Check sheet for the modelled part. Datum: model origin and axes. Units: mm. A direction names the side the tool comes from. Give positions to 0.01 mm unless a question says otherwise; leave off trailing zeros. Order: outer loops, then holes, each group sorted by start corner. A loop starts at its lowest first (then second) coordinate and runs counter-clockwise, first axis right, second up.
Item 1: Gauge pin test, flat ends, axial feed: P1, Ø8, axis at y = -17.5, z = -8, coming from the +X side; P2, Ø6, axis at x = 14, z = -8.5, coming from the -Y side; P3, Ø9, axis at y = -22, z = -4.5, coming from the -X side; P4, Ø12, axis at y = -4.5, z = -23.5, coming from the +X side. Record the tip position at first contact, or that the pin passes through.
Item 2: Material ranges on line 1 along X through (y, z) = (0.15, -20.25); line 2 along Z through (x, y) = (-21, -21.75); line 3 along Z through (x, y) = (-20, -7), recorded low to high.
Item 3: Release check for a two-part mould opening along Z. For faces 4 (the flat face through (-29, -6, -14.6)), 5 (the flat face through (11.719, -8, -48)), 6 (the flat face through (7.804, -5.144, -38.064)) record: released by +Z, released by -Z, zero draft, split by the parting line, or undercut.
Item 4: Sectioned sample at A-A on z = -9.5. Record the boundary of the cut face in (x, y), and give its area (3 significant figures).
Item 5: Sectioned sample at C-C on z = -15.5. Record the boundary of the cut face in (x, y), and give its area (3 significant figures).
Item 6: Access from +Z, -Z, +X, -X, +Y, -Y to the whole of each face (thin tool, end or side, straight path). Record for faces 1 (the flat face through (-3.889, -6, -43)), 2 (the cylindrical face through (-19.17, -16.55, -12.85)), 3 (the flat face through (7.62, -8.4, -48.9)).
Item 7: Sectioned sample at B-B on x = -7.5. Record the boundary of the cut face in (y, z).
from build123d import *

# Parameters (mm, degrees)
EXTRUDE_1_DEPTH     = 22
SKETCH_2_W          = 5
SKETCH_2_H          = 1.8
SKETCH_2_W_2        = 7
SKETCH_2_H_2        = 2.3
CUT_EXTRUDE_1_DEPTH = 4
CUT_EXTRUDE_2_DEPTH = 64.319089808
SKETCH_3_3_R        = 14
EXTRUDE_2_DEPTH     = 0.3
SKETCH_4_W          = 4.8
SKETCH_4_H          = 4.8
EXTRUDE_3_DEPTH     = 0.8
SKETCH_5_R          = 0.85
CUT_EXTRUDE_3_DEPTH = 63.897702188
SKETCH_6_W          = 11
SKETCH_6_H          = 3
CUT_EXTRUDE_4_DEPTH = 1
SKETCH_7_W          = 4.8
SKETCH_7_H          = 4.8
EXTRUDE_4_DEPTH     = 0.8
SKETCH_9_W          = 1.5
SKETCH_9_H          = 0.3
CUT_EXTRUDE_5_DEPTH = 10
EXTRUDE_5_DEPTH     = 8
EXTRUDE_6_DEPTH     = 0.3
EXTRUDE_7_DEPTH     = 5
EXTRUDE_8_DEPTH     = 0.3
SKETCH_14_R         = 0.65
SKETCH_14_W         = 12
SKETCH_14_H         = 2
CUT_EXTRUDE_6_DEPTH = 4
SKETCH_15_R         = 0.65
CUT_EXTRUDE_7_DEPTH = 4
SKETCH_16_R         = 0.65
CUT_EXTRUDE_8_DEPTH = 4


with BuildPart() as part:
    # Sketch 1 → Extrude 1 (new body)
    with BuildSketch(Plane(origin=(0, 0, 0), x_dir=(0, 0, -1), z_dir=(1, 0, 0))):
        with BuildLine():
            Line((0, -25), (0, -2))
            ThreePointArc((0, -2), (0.585786438, -0.585786438), (2, 0))
            Line((2, 0), (23.64572618, 0))
            ThreePointArc((23.64572618, 0), (23.99456936, -0.030657867), (24.332717753, -0.121691565))
            Line((24.332717753, -0.121691565), (52.174626532, -10.304873595))
            Line((52.174626532, -10.304873595), (52.277675268, -10.023127329))
            Line((52.277675268, -10.023127329), (24.435766489, 0.160054701))
            ThreePointArc((24.435766489, 0.160054701), (24.046895837, 0.264743453), (23.64572618, 0.3))
            Line((23.64572618, 0.3), (2, 0.3))
            ThreePointArc((2, 0.3), (0.373654403, -0.373654403), (-0.3, -2))
            Line((-0.3, -2), (-0.3, -25))
            Line((-0.3, -25), (0, -25))
        make_face()
    extrude(amount=EXTRUDE_1_DEPTH)

    # Sketch 2 → Cut-Extrude 1 (cut)
    with BuildSketch(Plane.XY.offset(0.3)):
        with Locations((8.5, -0.9)):
            Rectangle(SKETCH_2_W, SKETCH_2_H)
        with Locations((13.5, -0.9)):
            Rectangle(SKETCH_2_W, SKETCH_2_H)
        with Locations((7.5, -3.15)):
            Rectangle(SKETCH_2_W_2, SKETCH_2_H_2)
        with Locations((14.5, -3.15)):
            Rectangle(SKETCH_2_W_2, SKETCH_2_H_2)
        Polygon((4, -1.8), (4, -2), (11, -2), (11, -1.8), (6, -1.8), align=None)
        Polygon((11, -1.8), (11, -2), (18, -2), (18, -1.8), (16, -1.8), align=None)
    extrude(amount=-CUT_EXTRUDE_1_DEPTH, mode=Mode.SUBTRACT)

    # Sketch 3 → Cut-Extrude 2 (cut, through all)
    with BuildSketch(Plane(origin=(0, 8.024038665, -2.934793264), x_dir=(1, 0, 0), z_dir=(0, 0.9391542177229502, -0.3434957864853564))):
        with BuildLine():
            ThreePointArc((13.196152423, 52.539701225), (19.591939741, 47.38998358), (22, 39.539701225))
            Line((22, 39.539701225), (22, 52.539701225))
            Line((22, 52.539701225), (13.196152423, 52.539701225))
        make_face()
        with BuildLine():
            ThreePointArc((0, 51.028826518), (1.358818231, 51.864258204), (2.803847577, 52.539701225))
            Line((2.803847577, 52.539701225), (0, 52.539701225))
            Line((0, 52.539701225), (0, 51.028826518))
        make_face()
    extrude(amount=-CUT_EXTRUDE_2_DEPTH, mode=Mode.SUBTRACT)

    # Sketch 3_3 → Extrude 2 (add)
    with BuildSketch(Plane(origin=(0, 8.024038665, -2.934793264), x_dir=(1, 0, 0), z_dir=(0, 0.9391542177229502, -0.3434957864853564))):
        with Locations((8, 39.539701225)):
            Circle(SKETCH_3_3_R)
    extrude(amount=-EXTRUDE_2_DEPTH)

    # Sketch 4 → Extrude 3 (add)
    with BuildSketch(Plane.XY.offset(0.3)):
        with Locations((11, -9.75)):
            Rectangle(SKETCH_4_W, SKETCH_4_H)
        with Locations((11, -21.05)):
            Rectangle(SKETCH_4_W, SKETCH_4_H)
        with Locations((5.35, -15.4)):
            Rectangle(SKETCH_4_W, SKETCH_4_H)
        with Locations((16.65, -15.4)):
            Rectangle(SKETCH_4_W, SKETCH_4_H)
    extrude(amount=EXTRUDE_3_DEPTH)

    # Sketch 5 → Cut-Extrude 3 (cut, through all)
    with BuildSketch(Plane(origin=(0, 0.3, 0), x_dir=(1, 0, 0), z_dir=(0, 1, 0))):
        with Locations(Location((8, 6.64572618, 0), (0, 0, 270))):
            Circle(SKETCH_5_R)
        with Locations(Location((14, 6.64572618, 0), (0, 0, 270))):
            Circle(SKETCH_5_R)
    extrude(amount=-CUT_EXTRUDE_3_DEPTH, mode=Mode.SUBTRACT)

    # Sketch 6 → Cut-Extrude 4 (cut)
    with BuildSketch(Plane(origin=(0, 8.024038665, -2.934793264), x_dir=(1, 0, 0), z_dir=(0, 0.9391542177229502, -0.3434957864853564))):
        with Locations((11, 24.5)):
            Rectangle(SKETCH_6_W, SKETCH_6_H)
    extrude(amount=-CUT_EXTRUDE_4_DEPTH, mode=Mode.SUBTRACT)

    # Sketch 7 → Extrude 4 (add)
    with BuildSketch(Plane(origin=(0, 8.024038665, -2.934793264), x_dir=(1, 0, 0), z_dir=(0, 0.9391542177229502, -0.3434957864853564))):
        with Locations((9.738477049, 36.851443585)):
            Rectangle(SKETCH_7_W, SKETCH_7_H)
        with Locations((14.118767038, 47.774445204)):
            Rectangle(SKETCH_7_W, SKETCH_7_H)
        with Locations((5.219570287, 48.855656024)):
            Rectangle(SKETCH_7_W, SKETCH_7_H)
        with Locations((-1.489481468, 43.037611303)):
            Rectangle(SKETCH_7_W, SKETCH_7_H)
        with Locations((-1.651961899, 34.079108149)):
            Rectangle(SKETCH_7_W, SKETCH_7_H)
    extrude(amount=EXTRUDE_4_DEPTH)

    # Sketch 9 → Cut-Extrude 5 (cut)
    with BuildSketch(Plane.XZ.offset(25)):
        with Locations((0.75, 0.15)):
            Rectangle(SKETCH_9_W, SKETCH_9_H)
    extrude(amount=-CUT_EXTRUDE_5_DEPTH, mode=Mode.SUBTRACT)

    # Sketch 10 → Extrude 5 (add)
    with BuildSketch(Plane.XZ.offset(25)):
        with BuildLine():
            Line((1.5, 0), (1.4, 0))
            ThreePointArc((1.4, 0), (0.339339828, -0.439339828), (-0.1, -1.5))
            Line((-0.1, -1.5), (-0.1, -11.5))
            ThreePointArc((-0.1, -11.5), (-0.539339828, -12.560660172), (-1.6, -13))
            Line((-1.6, -13), (-17.6, -13))
            Line((-17.6, -13), (-17.6, -12.7))
            Line((-17.6, -12.7), (-1.6, -12.7))
            ThreePointArc((-1.6, -12.7), (-0.751471863, -12.348528137), (-0.4, -11.5))
            Line((-0.4, -11.5), (-0.4, -1.5))
            ThreePointArc((-0.4, -1.5), (0.127207794, -0.227207794), (1.4, 0.3))
            Line((1.4, 0.3), (1.5, 0.3))
            Line((1.5, 0.3), (1.5, 0))
        make_face()
    extrude(amount=-EXTRUDE_5_DEPTH)

    # Sketch 11 → Extrude 6 (add)
    with BuildSketch(Plane.XY.offset(-12.7)):
        with BuildLine():
            Line((-17.6, -17), (-17.6, -25))
            Line((-17.6, -25), (-23.1, -25))
            ThreePointArc((-23.1, -25), (-24.160660172, -24.560660172), (-24.6, -23.5))
            Line((-24.6, -23.5), (-24.6, -11))
            Line((-24.6, -11), (-19.6, -11))
            Line((-19.6, -11), (-19.6, -15.5))
            ThreePointArc((-19.6, -15.5), (-19.160660172, -16.560660172), (-18.1, -17))
            Line((-18.1, -17), (-17.6, -17))
        make_face()
    extrude(amount=-EXTRUDE_6_DEPTH)

    # Sketch 12 → Extrude 7 (add)
    with BuildSketch(Plane.ZY.offset(24.6)):
        with BuildLine():
            Line((-13, -11), (-13, -10.831371462))
            ThreePointArc((-13, -10.831371462), (-13.188036278, -10.104218664), (-13.70500159, -9.559374006))
            Line((-13.70500159, -9.559374006), (-13.89499841, -9.440625994))
            ThreePointArc((-13.89499841, -9.440625994), (-14.411963722, -8.895781336), (-14.6, -8.168628538))
            Line((-14.6, -8.168628538), (-14.6, -8))
            Line((-14.6, -8), (-14.3, -8))
            Line((-14.3, -8), (-14.3, -8.168628538))
            ThreePointArc((-14.3, -8.168628538), (-14.149570977, -8.750350777), (-13.735998728, -9.186226503))
            Line((-13.735998728, -9.186226503), (-13.546001908, -9.304974515))
            ThreePointArc((-13.546001908, -9.304974515), (-12.925643534, -9.958788104), (-12.7, -10.831371462))
            Line((-12.7, -10.831371462), (-12.7, -11))
            Line((-12.7, -11), (-13, -11))
        make_face()
    extrude(amount=-EXTRUDE_7_DEPTH)

    # Sketch 13 → Extrude 8 (add)
    with BuildSketch(Plane.XY.offset(-14.3)):
        with BuildLine():
            Line((-24.6, -8), (-19.6, -8))
            Line((-19.6, -8), (-19.6, -4.1))
            ThreePointArc((-19.6, -4.1), (-19.775735931, -3.675735931), (-20.2, -3.5))
            Line((-20.2, -3.5), (-34, -3.5))
            ThreePointArc((-34, -3.5), (-34.424264069, -3.675735931), (-34.6, -4.1))
            Line((-34.6, -4.1), (-34.6, -11))
            Line((-34.6, -11), (-28.1, -11))
            Line((-28.1, -11), (-28.1, -6.8))
            ThreePointArc((-28.1, -6.8), (-27.924264069, -6.375735931), (-27.5, -6.2))
            Line((-27.5, -6.2), (-25.2, -6.2))
            ThreePointArc((-25.2, -6.2), (-24.775735931, -6.375735931), (-24.6, -6.8))
            Line((-24.6, -6.8), (-24.6, -8))
        make_face()
    extrude(amount=-EXTRUDE_8_DEPTH)

    # Sketch 14 → Cut-Extrude 6 (cut)
    with BuildSketch(Plane(origin=(0, 8.024038665, -2.934793264), x_dir=(1, 0, 0), z_dir=(0, 0.9391542177229502, -0.3434957864853564))):
        with Locations(Location((0.5, 47.950575932, 0), (0, 0, 270))):
            Circle(SKETCH_14_R)
        with Locations(Location((19.5, 32.450575932, 0), (0, 0, 270))):
            Circle(SKETCH_14_R)
        with Locations((8, 53.550575932)):
            Rectangle(SKETCH_14_W, SKETCH_14_H)
    extrude(amount=-CUT_EXTRUDE_6_DEPTH, mode=Mode.SUBTRACT)

    # Sketch 15 → Cut-Extrude 7 (cut)
    with BuildSketch(Plane(origin=(0, 0.3, 0), x_dir=(1, 0, 0), z_dir=(0, 1, 0))):
        with Locations(Location((2.8, 20.25, 0), (0, 0, 270))):
            Circle(SKETCH_15_R)
        with Locations(Location((2.8, 7.25, 0), (0, 0, 270))):
            Circle(SKETCH_15_R)
        with Locations(Location((19.2, 7.25, 0), (0, 0, 270))):
            Circle(SKETCH_15_R)
    extrude(amount=-CUT_EXTRUDE_7_DEPTH, mode=Mode.SUBTRACT)

    # Sketch 16 → Cut-Extrude 8 (cut)
    with BuildSketch(Plane.XY.offset(0.3)):
        with Locations((19, -6)):
            Circle(SKETCH_16_R)
        with Locations((4, -23)):
            Circle(SKETCH_16_R)
    extrude(amount=-CUT_EXTRUDE_8_DEPTH, mode=Mode.SUBTRACT)


solid = part.part
Report:
1. P1: stops at x = -0.1
1. P2: stops at y = 0
1. P3: stops at x = -0.4
1. P4: stops at x = 22
2. line 1: x = 0 to 2.15, 3.45 to 22
2. line 2: z = -13 to -12.7
2. line 3: z = -14.6 to -14.3
3. face 4: released by -Z
3. face 5: zero draft
3. face 6: undercut
4. outline: (-0.4, -25) - (-0.1, -25) - (-0.1, -17) - (-0.4, -17) - close; (0, 0) - (22, 0) - (22, 0.3) - (0, 0.3) - close
4. area: 9.00 mm2
5. outline: (0, 0) - (22, 0) - (22, 0.3) - (0, 0.3) - close
5. area: 6.60 mm2
6. face 1: -Z, -X, +Y
6. face 2: +Z, -Z, +X, +Y
6. face 3: -Z, +Y
7. outline: (-25, -13) - (-17, -13) - (-17, -12.7) - (-25, -12.7) - close
